```python
from build123d import *

# Parameters (mm, degrees)
SKETCH1_R           = 35
SKETCH1_R_2         = 4.175
BOSS_EXTRUDE1_DEPTH = 2.5
SKETCH1_3_R         = 42.5
SKETCH1_3_R_2       = 35
BOSS_EXTRUDE2_DEPTH = 7.5
SKETCH2_R           = 8
BOSS_EXTRUDE3_DEPTH = 13
FILLET1_R           = 4
SKETCH3_R           = 1.5
CUT_EXTRUDE1_DEPTH  = 12.5


with BuildPart() as part:
    # Sketch1 → Boss-Extrude1 (new, symmetric)
    with BuildSketch(Plane(origin=(0, 0, 0), x_dir=(1, 0, 0), z_dir=(0, 1, 0))):
        with Locations(Location((0, 0, 0), (0, 0, 270))):
            Circle(SKETCH1_R)
        with Locations(Location((0, 0, 0), (0, 0, 270))):
            Circle(SKETCH1_R_2, mode=Mode.SUBTRACT)
    extrude(amount=BOSS_EXTRUDE1_DEPTH, both=True)

    # Sketch1_3 → Boss-Extrude2 (add, symmetric)
    with BuildSketch(Plane(origin=(0, 0, 0), x_dir=(1, 0, 0), z_dir=(0, 1, 0))):
        with Locations(Location((0, 0, 0), (0, 0, 270))):
            Circle(SKETCH1_3_R)
        with Locations(Location((0, 0, 0), (0, 0, 270))):
            Circle(SKETCH1_3_R_2, mode=Mode.SUBTRACT)
    extrude(amount=BOSS_EXTRUDE2_DEPTH, both=True)

    # Sketch2 → Boss-Extrude3 (add)
    with BuildSketch(Plane(origin=(0, 2.5, 0), x_dir=(1, 0, 0), z_dir=(0, 1, 0))):
        with Locations(Location((0, 0, 0), (0, 0, 90))):
            Circle(SKETCH2_R)
        with BuildLine():
            Line((-2.744966985, 3.1125), (2.744966985, 3.1125))
            ThreePointArc((2.744966985, 3.1125), (0, -4.15), (-2.744966985, 3.1125))
        make_face(mode=Mode.SUBTRACT)
    extrude(amount=BOSS_EXTRUDE3_DEPTH)

    # Fillet1
    fillet1_edges = [part.edges().sort_by_distance(p)[0] for p in [
        (0, 2.5, 8),
    ]]
    fillet(fillet1_edges, radius=FILLET1_R)

    # Sketch3 → Cut-Extrude1 (cut, symmetric)
    with BuildSketch(Plane.XY):
        with Locations(Location((0, 10, 0), (0, 0, 90))):
            Circle(SKETCH3_R)
    extrude(amount=CUT_EXTRUDE1_DEPTH, both=True, mode=Mode.SUBTRACT)


solid = part.part
```
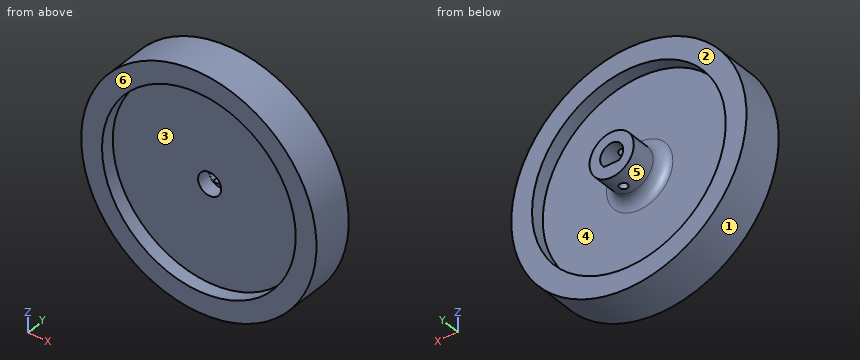
Source: CAD feature listing. Evaluate the final solid. Frame: model axes, mm. Face numbers are marked on the shaded views. A direction names the side the tool comes from. Round coordinates to 2 decimals unless told otherwise and drop trailing zeros. Loops run counter-clockwise (first coordinate to the right, second up) from the corner with the lowest first, then second, coordinate; pieces in that order, holes last.
(1) Pull-direction query (X, two-part tool) for the marked faces 1, 2, 3 and 4; classes: +X half, -X half, draft (parallel to the pull), parting line (faces both ways), or undercut.
From the geometry:
face 1: parting line
face 2: draft
face 3: undercut
face 4: undercut
(2) Section query B-B (y = 4.5). Output: boundary loops of the cut face in (x, z), and give its area (3 significant figures).
From the geometry:
outline: circle Ø85 at (0, 0); circle Ø17.07 at (0, 0); hole circle Ø70 at (0, 0); hole (-2.74, -3.11) - (2.74, -3.11) arc R4.15 ccw (long way) to start
area: 2,000 mm2
(3) Contact query for flat-ended pins moving along their axis: pin 1 Ø2.5 at (x, y) = (1, 8.5) entering from +Z; pin 2 Ø3 at (x, z) = (11.5, 22) entering from -Y; pin 3 Ø2 at (x, y) = (-2.5, 12.5) entering from +Z; pin 4 Ø5 at (x, z) = (0, 0) entering from +Y. Output: stop coordinate, or through.
From the geometry:
pin 1: stops at z = 42.5
pin 2: stops at y = -2.5
pin 3: stops at z = 7.86
pin 4: passes through
(4) Material intervals for probe 1 along X at (y, z) = (4, 0); probe 2 along X at (y, z) = (1.15, 0) (3 decimals); probe 3 along Y at (x, z) = (30.5, 13), sorted ascending.
From the geometry:
probe 1: x = -42.5 to -35, -8.88 to -4.15, 4.15 to 8.88, 35 to 42.5
probe 2: x = -42.5 to -4.175, 4.175 to 42.5
probe 3: y = -2.5 to 2.5
(5) Section query A-A (x = 0). Give the number of separate pieces and of enclosed holes in the cut face, and give its area (3 significant figures).
From the geometry:
separate pieces: 4
enclosed holes: 0
area: 627 mm2
(6) Access query for the marked faces 5 and 6. Directions: +Z, -Z, +X, -X, +Y, -Y. A direction counts if a zero-diameter tool reaches every point of the face in a straight line with its end or side. Return the directions, or none.
From the geometry:
face 5: +Y
face 6: +Z, -Z, +X, -X, -Y
(7) Section query C-C (z = 0). Output: boundary loops of the cut face in (x, y) (3 decimals).
From the geometry:
outline: (-42.5, -7.5) - (-35, -7.5) - (-35, -2.5) - (-4.175, -2.5) - (-4.175, 2.5) - (-4.15, 2.5) - (-4.15, 15.5) - (-8, 15.5) - (-8, 6.5) arc R4 cw to (-12, 2.5) - (-35, 2.5) - (-35, 7.5) - (-42.5, 7.5) - close; (4.15, 2.5) - (4.175, 2.5) - (4.175, -2.5) - (35, -2.5) - (35, -7.5) - (42.5, -7.5) - (42.5, 7.5) - (35, 7.5) - (35, 2.5) - (12, 2.5) arc R4 cw to (8, 6.5) - (8, 15.5) - (4.15, 15.5) - close
(8) Section query D-D (y = 10). Output: boundary loops of the cut face in (x, z).
From the geometry:
outline: (-2.74, -3.11) arc R4.15 cw to (-1.5, 3.87) - (-1.5, 7.86) arc R8 ccw to (-1.5, -7.86) - (-1.5, -3.11) - close; (1.5, -7.86) arc R8 ccw to (1.5, 7.86) - (1.5, 3.87) arc R4.15 cw to (2.74, -3.11) - (1.5, -3.11) - close
